Design review of the part built by this model. Coordinates are the model's own, in mm. A direction names the side the tool comes from. Coordinates: 2 decimals unless noted, no trailing zeros. Loops run counter-clockwise (first coordinate to the right, second up) from the corner with the lowest first, then second, coordinate; pieces in that order, holes last. Notation, with made-up numbers: (24, 54) -> (80, 54) arc R32 cw to (80, 84) -> close; hole circle Ø4 at (46, 9). An arc over 180 degrees is marked (long way). Use a Markdown table: item, result. Add a question column.
Q1. Take a section at B-B on x = 0. Write out the cut boundary in (y, z).
Q2. Clearance check with flat-ended pins moving along their axes: pin 1 Ø2 at (x, y) = (-7, 9) entering from -Z; pin 2 Ø2 at (x, y) = (-6.5, 7.5) entering from +Z. State where each tip first meets the part, or that it passes through.
Q3. Take a section at A-A on z = 0. Write out the cut boundary in (x, y).
Q4. Take a section at C-C on y = 7.2. Write out the cut boundary in (x, z).
Q5. Draft analysis for pull direction Z (two halves, no side actions). For faces 1 (the face through (-5, 11.857, 8)), 2 (the face through (-0.33, 7.35, 7.493)), 3 (the face through (-3.2, 9.3, -10)), 4 (the face through (-2.703, 11.364, -8.584)), state which applies: pulls with the +Z half, pulls with the -Z half, needs draft (parallel to the pull), parting line crosses it, or undercut.
Q6. For probe 1 along X at (y, z) = (11.4, 0); probe 2 along X at (y, z) = (7.5, -3.5); probe 3 along X at (y, z) = (7.2, 6.25), list the stretches that pass through material, from the lowest coordinate up.
Q7. Take a section at D-D on z = -6.25. Write out the cut boundary in (x, y), plus the area to 3 significant figures.
Q8. For faces 5 (the face through (-5, 6.857, -8)), 6 (the face through (-0.33, 11.35, 7.493)), 7 (the face through (-7.4, 7.857, 2)), list the 3-axis set-ups (+Z, -Z, +X, -X, +Y, -Y) from which the entire face can be reached by the end or side of a thin tool; tool diameter is ignored.
from build123d import *


with BuildPart() as part:
    # Croquis1 → Revolución1 (revolve)
    with BuildSketch(Plane.XY, mode=Mode.PRIVATE) as revoluci_n1_sk:
        Polygon((-6, 6.856705357), (-6, 11.856705357), (-7.5, 11.856705357), (-7.5, 10.856705357), (-9, 10.856705357), (-9, 11.856705357), (-10.5, 11.856705357), (-10.5, 6.856705357), (-9, 6.856705357), (-9, 7.856705357), (-7.5, 7.856705357), (-7.5, 6.856705357), align=None)
    revolve(revoluci_n1_sk.sketch.rotate(Axis((0, 0, 0), (0, 1, 0)), 270), axis=Axis((0, 0, 0), (0, 1, 0)))


solid = part.part
Answer list:
| question | item | result |
|---|---|---|
| 1 | outline | (6.86, -10.5) -> (11.86, -10.5) -> (11.86, -9) -> (10.86, -9) -> (10.86, -7.5) -> (11.86, -7.5) -> (11.86, -6) -> (6.86, -6) -> (6.86, -7.5) -> (7.86, -7.5) -> (7.86, -9) -> (6.86, -9) -> close; (6.86, 6) -> (11.86, 6) -> (11.86, 7.5) -> (10.86, 7.5) -> (10.86, 9) -> (11.86, 9) -> (11.86, 10.5) -> (6.86, 10.5) -> (6.86, 9) -> (7.86, 9) -> (7.86, 7.5) -> (6.86, 7.5) -> close |
| 2 | pin 1 | z = -8.62 |
| 2 | pin 2 | z = 8.94 |
| 3 | outline | (-10.5, 6.86) -> (-9, 6.86) -> (-9, 7.86) -> (-7.5, 7.86) -> (-7.5, 6.86) -> (-6, 6.86) -> (-6, 11.86) -> (-7.5, 11.86) -> (-7.5, 10.86) -> (-9, 10.86) -> (-9, 11.86) -> (-10.5, 11.86) -> close; (6, 6.86) -> (7.5, 6.86) -> (7.5, 7.86) -> (9, 7.86) -> (9, 6.86) -> (10.5, 6.86) -> (10.5, 11.86) -> (9, 11.86) -> (9, 10.86) -> (7.5, 10.86) -> (7.5, 11.86) -> (6, 11.86) -> close |
| 4 | outline | circle Ø21 at (0, 0); circle Ø15 at (0, 0); hole circle Ø18 at (0, 0); hole circle Ø12 at (0, 0) |
| 5 | face 1 | needs draft |
| 5 | face 2 | undercut |
| 5 | face 3 | parting line crosses it |
| 5 | face 4 | undercut |
| 6 | probe 1 | -10.5 to -9, -7.5 to -6, 6 to 7.5, 9 to 10.5 |
| 6 | probe 2 | -9.9 to -8.29, -6.63 to -4.87, 4.87 to 6.63, 8.29 to 9.9 |
| 6 | probe 3 | -8.44 to -6.48, -4.15 to 4.15, 6.48 to 8.44 |
| 7 | outline | (-8.44, 6.86) -> (-6.48, 6.86) -> (-6.48, 7.86) -> (-4.15, 7.86) -> (-4.15, 6.86) -> (4.15, 6.86) -> (4.15, 7.86) -> (6.48, 7.86) -> (6.48, 6.86) -> (8.44, 6.86) -> (8.44, 11.86) -> (6.48, 11.86) -> (6.48, 10.86) -> (4.15, 10.86) -> (4.15, 11.86) -> (-4.15, 11.86) -> (-4.15, 10.86) -> (-6.48, 10.86) -> (-6.48, 11.86) -> (-8.44, 11.86) -> close |
| 7 | area | 75.1 mm² |
| 8 | face 5 | +Z, -Z, +X, -X, -Y |
| 8 | face 6 | +Y |
| 8 | face 7 | -Y |
